Source: CAD feature listing. Evaluate the final solid. Frame: model axes, mm. A direction names the side the tool comes from. Round coordinates to 2 decimals unless told otherwise and drop trailing zeros. Order: outer loops, then holes, each group sorted by start corner. A loop starts at its lowest first (then second) coordinate and runs counter-clockwise, first axis right, second up. Notation, with made-up numbers: (20, 28) -> (36, 28) arc R19 cw to (36, 38) -> close; hole circle Ø7 at (53, -30.5). An arc over 180 degrees is marked (long way). Answer as CSV lines item,"result".
from build123d import *

# Parameters (mm, degrees)
SKETCH2_W           = 7
SKETCH2_H           = 13
SKETCH2_R           = 1.25
BOSS_EXTRUDE1_DEPTH = 5
FILLET1_R           = 1
SKETCH3_R           = 0.7
CUT_EXTRUDE1_DEPTH  = 3


with BuildPart() as part:
    # Sketch2 → Boss-Extrude1 (new body)
    with BuildSketch(Plane.XY):
        Rectangle(SKETCH2_W, SKETCH2_H)
        with Locations((0, 4.5)):
            Circle(SKETCH2_R, mode=Mode.SUBTRACT)
        with Locations((0, 1.5)):
            Circle(SKETCH2_R, mode=Mode.SUBTRACT)
        with Locations((0, -1.5)):
            Circle(SKETCH2_R, mode=Mode.SUBTRACT)
        with Locations((0, -4.5)):
            Circle(SKETCH2_R, mode=Mode.SUBTRACT)
    extrude(amount=BOSS_EXTRUDE1_DEPTH)

    # Fillet1
    fillet1_edges = [part.edges().sort_by_distance(p)[0] for p in [
        (-3.5, 0, 0),
        (3.5, 0, 0),
        (3.5, 0, 5),
        (-3.5, 0, 5),
    ]]
    fillet(fillet1_edges, radius=FILLET1_R)

    # Sketch3 → Cut-Extrude1 (cut)
    with BuildSketch(Plane(origin=(0, 6.5, 0), x_dir=(1, 0, 0), z_dir=(0, 1, 0))):
        with Locations((-2, -2.5)):
            Circle(SKETCH3_R)
        with Locations((2, -2.5)):
            Circle(SKETCH3_R)
    cut_extrude1 = extrude(amount=-CUT_EXTRUDE1_DEPTH, mode=Mode.SUBTRACT)

    # Mirror1: Cut-Extrude1 across plane
    add(cut_extrude1.mirror(Plane.ZX), mode=Mode.SUBTRACT)


solid = part.part
1. Section query A-A on y = 4.5. Return loops of the section in (x, z).
Results below:
outline,"(-3.5, 1) arc R1 ccw to (-2.5, 0) -> (-1.25, 0) -> (-1.25, 5) -> (-2.5, 5) arc R1 ccw to (-3.5, 4) -> close; (1.25, 0) -> (2.5, 0) arc R1 ccw to (3.5, 1) -> (3.5, 4) arc R1 ccw to (2.5, 5) -> (1.25, 5) -> close; hole circle Ø1.4 at (-2, 2.5); hole circle Ø1.4 at (2, 2.5)"
2. Section query B-B on x = 0. Return loops of the section in (y, z), and give its area (3 significant figures).
Results below:
outline,"(-6.5, 0) -> (-5.75, 0) -> (-5.75, 5) -> (-6.5, 5) -> close; (-3.25, 0) -> (-2.75, 0) -> (-2.75, 5) -> (-3.25, 5) -> close; (-0.25, 0) -> (0.25, 0) -> (0.25, 5) -> (-0.25, 5) -> close; (2.75, 0) -> (3.25, 0) -> (3.25, 5) -> (2.75, 5) -> close; (5.75, 0) -> (6.5, 0) -> (6.5, 5) -> (5.75, 5) -> close"
area,"15.0 mm2"
3. Line query: L1, parallel to Y at x = 0, z = 3.25; L2, parallel to Z at x = 2, y = 5.3; L3, parallel to Y at x = 0.75, z = 2.3. Output: solid intervals per line, ascending. Write a range as [from, to].
Results below:
L1,"[-6.5, -5.75], [-3.25, -2.75], [-0.25, 0.25], [2.75, 3.25], [5.75, 6.5]"
L2,"[0, 1.8], [3.2, 5]"
L3,"[-6.5, -5.5], [-3.5, -2.5], [-0.5, 0.5], [2.5, 3.5], [5.5, 6.5]"
4. Mould query, pull axis Y, two halves, no side actions, for faces 4 (the cylindrical face through (-0.27, 0.28, 2.46)), 5 (the flat face through (-2, 3.5, 2)), 6 (the cylindrical face through (-1.353, 5.021, 2.768)). Classes: released by +Y, released by -Y, zero draft, split by the parting line, or undercut.
Results below:
face 4,"undercut"
face 5,"released by +Y"
face 6,"zero draft"
5. Section query D-D on y = -1.5. Return loops of the section in (x, z), and give its area (3 significant figures).
Results below:
outline,"(-3.5, 1) arc R1 ccw to (-2.5, 0) -> (-1.25, 0) -> (-1.25, 5) -> (-2.5, 5) arc R1 ccw to (-3.5, 4) -> close; (1.25, 0) -> (2.5, 0) arc R1 ccw to (3.5, 1) -> (3.5, 4) arc R1 ccw to (2.5, 5) -> (1.25, 5) -> close"
area,"21.6 mm2"
6. Reachability of faces 1 (the cylindrical face through (1.848, -5.021, 3.183)), 2 (the cylindrical face through (-3.215, 0.091, 0.301)), 3 (the cylindrical face through (1.848, 5.021, 3.183)) from +Z, -Z, +X, -X, +Y, -Y: full face, straight path, thin tool, end or side. Return the list, or none.
Results below:
face 1,"-Y"
face 2,"-Z, -X, +Y, -Y"
face 3,"+Y"
7. Pin query (flat end, axial travel): pin 1 (1.1 mm diameter, centred on x = 2, z = 2.5, fed in from +Y); pin 2 (1.1 mm diameter, centred on x = -2, z = 2.5, fed in from -Y). Return the tip coordinate at first contact, or that it passes through.
Results below:
pin 1,"y = 3.5"
pin 2,"y = -3.5"
8. Section query C-C on z = 3.6. Return loops of the section in (x, y), and give its area (3 significant figures).
Results below:
outline,"(-3.5, -6.5) -> (3.5, -6.5) -> (3.5, 6.5) -> (-3.5, 6.5) -> close; hole circle Ø2.5 at (0, -4.5); hole circle Ø2.5 at (0, -1.5); hole circle Ø2.5 at (0, 1.5); hole circle Ø2.5 at (0, 4.5)"
area,"71.4 mm2"
